CAD build for the part. Positions are in the model's coordinates, mm. A direction names the side the tool comes from. Round coordinates to 2 decimals unless told otherwise and drop trailing zeros. Loops run counter-clockwise (first coordinate to the right, second up) from the corner with the lowest first, then second, coordinate; pieces in that order, holes last. Notation, with made-up numbers: (-1.5, -26) -> (29.5, -26) arc R21 ccw to (29.5, 12) -> close; hole circle Ø1 at (22.25, 9.5). An arc over 180 degrees is marked (long way). Answer as CSV lines item,"result".
```python
from build123d import *

# Parameters (mm, degrees)
BOSS_EXTRUDE1_DEPTH = 6.35
SKETCH2_R           = 2.54
BOSS_EXTRUDE2_DEPTH = 19.05
SKETCH3_R           = 2.54
CUT_EXTRUDE1_DEPTH  = 19.05


with BuildPart() as part:
    # Sketch1 → Boss-Extrude1 (new, symmetric)
    with BuildSketch(Plane.XY):
        with BuildLine():
            Line((0, -53.34), (19.05, -53.34))
            Line((19.05, -53.34), (19.05, -50.501466563))
            ThreePointArc((19.05, -50.501466563), (44.393267367, -30.700788874), (53.975, 0))
            Line((53.975, 0), (50.8, 0))
            ThreePointArc((50.8, 0), (0, -50.8), (-50.8, 0))
            Line((-50.8, 0), (-54.0004, 0))
            ThreePointArc((-54.0004, 0), (-44.411433326, -30.71917626), (-19.05, -50.528612688))
            Line((-19.05, -50.528612688), (-19.05, -53.34))
            Line((-19.05, -53.34), (0, -53.34))
        make_face()
    extrude(amount=BOSS_EXTRUDE1_DEPTH, both=True)

    # Sketch2 → Boss-Extrude2 (add)
    with BuildSketch(Plane(origin=(50.8, 0, 0), x_dir=(0, 0, -1), z_dir=(1, 0, 0))):
        with BuildLine():
            Line((-6.35, 0), (6.35, 0))
            Line((6.35, 0), (6.35, 4.318))
            Line((6.35, 4.318), (4.318, 4.318))
            ThreePointArc((4.318, 4.318), (0, 8.636), (-4.318, 4.318))
            Line((-4.318, 4.318), (-6.35, 4.318))
            Line((-6.35, 4.318), (-6.35, 0))
        make_face()
        with Locations(Location((0, 4.318, 0), (0, 0, 180))):
            Circle(SKETCH2_R, mode=Mode.SUBTRACT)
    boss_extrude2 = extrude(amount=BOSS_EXTRUDE2_DEPTH)

    # Mirror1: Boss-Extrude2 across plane
    add(boss_extrude2.mirror(Plane(origin=(0, 0, 0), x_dir=(0, 0, 1), z_dir=(1, 0, 0))))

    # Sketch3 → Cut-Extrude1 (cut)
    with BuildSketch(Plane.XZ.offset(53.34)):
        with Locations(Location((-9.525, 0, 0), (0, 0, 270))):
            Circle(SKETCH3_R)
        with Locations(Location((9.525, 0, 0), (0, 0, 270))):
            Circle(SKETCH3_R)
    extrude(amount=-CUT_EXTRUDE1_DEPTH, mode=Mode.SUBTRACT)


solid = part.part
```
Q1. Slice it at C-C, the plane x = 0. Give the cut face in (y, z), and give its area (3 significant figures).
Results:
outline,"(-53.34, -6.35) -> (-50.8, -6.35) -> (-50.8, 6.35) -> (-53.34, 6.35) -> close"
area,"32.3 mm2"
Q2. Two-plate mould, pull along X, no slides. Class faces 1 (the flat face through (-50.8, 1, 0)), 2 (the flat face through (-69.85, 1, 0)), 3 (the cylindrical face through (60.192, 8.635, -0.095)): pulls with the +X half, pulls with the -X half, needs draft (parallel to the pull), parting line crosses it, or undercut.
Results:
face 1,"undercut"
face 2,"pulls with the -X half"
face 3,"needs draft"
Q3. Slice it at B-B, the plane y = -39. Give the cut face in (x, z), and give its area (3 significant figures).
Results:
outline,"(-37.35, -6.35) -> (-32.55, -6.35) -> (-32.55, 6.35) -> (-37.35, 6.35) -> close; (32.55, -6.35) -> (37.31, -6.35) -> (37.31, 6.35) -> (32.55, 6.35) -> close"
area,"121 mm2"
Q4. Probe L1, parallel to X at y = -51.6, z = 0 (3 decimals); L2, parallel to Y at x = 62, z = 0; L3, parallel to X at y = -0.5, z = 4.5. List the from-to ranges inside material, lowest first. Write a range as [from, to].
Results:
L1,"[-19.05, -12.065], [-6.985, 6.985], [12.065, 19.05]"
L2,"[0, 1.78], [6.86, 8.64]"
L3,"[-54, -50.8], [50.8, 53.97]"
Q5. Drop flat-ended pins along their axis: pin 1 Ø0.6 at (x, z) = (59.5, 5) entering from +Y; pin 2 Ø1.4 at (y, z) = (-52.5, -2.5) entering from -X; pin 3 Ø1.5 at (y, z) = (-10.5, 4.5) entering from -X. Give the stop position or say it passes through.
Results:
pin 1,"y = 4.32"
pin 2,"x = -19.05"
pin 3,"x = -53.11"
Q6. Slice it at A-A, the plane y = -5. Give the cut face in (x, z), and give its area (3 significant figures).
Results:
outline,"(-53.77, -6.35) -> (-50.55, -6.35) -> (-50.55, 6.35) -> (-53.77, 6.35) -> close; (50.55, -6.35) -> (53.74, -6.35) -> (53.74, 6.35) -> (50.55, 6.35) -> close"
area,"81.3 mm2"
Q7. Tool access for faces 4 (the flat face through (-10, -50, 6.35)), 5 (the flat face through (-62, 0, 0)), 6 (the flat face through (19.05, -52, 0)): list every direction of +Z, -Z, +X, -X, +Y, -Y with a clear straight run to the whole face (end or side of a thin tool).
Results:
face 4,"+Z, +X, -X, +Y, -Y"
face 5,"+Z, -Z, -X, -Y"
face 6,"+Z, -Z, +X, -Y"
Q8. Slice it at D-D, the plane x = 42.5. Give the cut face in (y, z), and give its area (3 significant figures).
Results:
outline,"(-33.27, -6.35) -> (-27.83, -6.35) -> (-27.83, 6.35) -> (-33.27, 6.35) -> close"
area,"69.1 mm2"
